```python
from build123d import *

# Parameters (mm, degrees)
BASE_FLANGE1_DEPTH           = 6.35
EDGE_FLANGE1_STRIP_W         = 41.3004
EDGE_FLANGE1_STRIP_H         = 6.35
EDGE_FLANGE1_STRIP_CUT_DEPTH = 520.7
EDGE_FLANGE1_DEPTH           = 520.7


# Sheet-metal steps are written as plain solids
with BuildPart() as part:
    # Sketch1 → Base-Flange1 (new body)
    with BuildSketch(Plane.XY):
        Polygon((-260.35, 127), (260.35, 127), (260.35, 46.0375), (269.875, 46.0375), (269.875, 20.6375), (260.35, 20.6375), (260.35, -112.7125), (269.875, -112.7125), (269.875, -138.1125), (215.9, -138.1125), (215.9, 0), (-215.9, 0), (-215.9, -138.1125), (-269.875, -138.1125), (-269.875, -112.7125), (-260.35, -112.7125), (-260.35, 20.6375), (-269.875, 20.6375), (-269.875, 46.0375), (-260.35, 46.0375), align=None)
    extrude(amount=-BASE_FLANGE1_DEPTH)

    # Edge-Flange1 strip (across the edge) → Edge-Flange1 strip cut (cut)
    with BuildSketch(Plane(origin=(260.35, 127, 0), x_dir=(0, -1, 0), z_dir=(-1, 0, 0))):
        with Locations((-6.35, -3.175)):
            Rectangle(EDGE_FLANGE1_STRIP_W, EDGE_FLANGE1_STRIP_H)
    extrude(amount=EDGE_FLANGE1_STRIP_CUT_DEPTH, mode=Mode.SUBTRACT)

    # Edge-Flange1 section (across the edge) → Edge-Flange1 (add)
    with BuildSketch(Plane(origin=(260.35, 127, 0), x_dir=(0, -1, 0), z_dir=(-1, 0, 0))):
        with BuildLine():
            Line((0, 7.9502), (0, 31.75))
            Line((0, 31.75), (6.35, 31.75))
            Line((6.35, 31.75), (6.35, 7.9502))
            ThreePointArc((6.35, 7.9502), (8.678559668, 2.328559668), (14.3002, 0))
            Line((14.3002, 0), (14.3002, -6.35))
            ThreePointArc((14.3002, -6.35), (4.188431608, -2.161568392), (0, 7.9502))
        make_face()
    extrude(amount=EDGE_FLANGE1_DEPTH)


solid = part.part
```
Build history of the part. All positions in model axes, mm. A direction names the side the tool comes from. Give positions to 0.01 mm unless a question says otherwise; leave off trailing zeros. Loops run counter-clockwise (first coordinate to the right, second up) from the corner with the lowest first, then second, coordinate; pieces in that order, holes last. Notation, with made-up numbers: (82.25, 51) -> (141.25, 51) arc R13 cw to (141.25, 61) -> close; hole circle Ø11 at (2.25, 72.25). An arc over 180 degrees is marked (long way). One line per question, with ' | ' between items. Start each with the question number.
1) 3-axis set-ups, long thin cutter, end or side, ignore diameter. For faces 1 (the flat face through (4, 120.65, 20)), 2 (the flat face through (-260.35, 98, -1)), 3 (the flat face through (260.35, 98, -1)): which of +Z, -Z, +X, -X, +Y, -Y reach the whole face in a straight line?
2) Cut at C-C (z = 14). Give the cut face in (x, y).
3) Probe L1, parallel to X at y = -104, z = -2; L2, parallel to Y at x = 79, z = 9; L3, parallel to Z at x = 117, y = 63. List the from-to ranges inside material, lowest first.
4) Cut at B-B (x = 13). Give the cut face in (y, z).
5) Cut at D-D (y = 33). Give the cut face in (x, z) (3 decimals).
6) Cut at A-A (y = -19). Give the cut face in (x, z), plus the area to 3 significant figures.
7) Two-plate mould, pull along Z, no slides. Class faces 4 (the flat face through (4, 45, -6.35)), 5 (the flat face through (4, 45, 0)), 6 (the flat face through (4, 127, 20)): released by +Z, released by -Z, zero draft, split by the parting line, or undercut.
8) Pin check, flat tips, straight feed: pin 1 (12 mm diameter, centred on x = 27, z = 14.5, fed in from -Y); pin 2 (3 mm diameter, centred on x = 267, z = -2, fed in from +Y); pin 3 (7 mm diameter, centred on x = 93, z = -2, fed in from -Y). Stop position of each tip, or through.
Return value:
1) face 1: +Z, +X, -X, -Y | face 2: +Z, -Z, -X, +Y | face 3: +Z, -Z, +X, +Y
2) outline: (-260.35, 120.65) -> (260.35, 120.65) -> (260.35, 127) -> (-260.35, 127) -> close
3) L1: -260.35 to -215.9, 215.9 to 260.35 | L2: 120.65 to 127 | L3: -6.35 to 0
4) outline: (0, -6.35) -> (112.7, -6.35) arc R14.3 ccw to (127, 7.95) -> (127, 31.75) -> (120.65, 31.75) -> (120.65, 7.95) arc R7.95 cw to (112.7, 0) -> (0, 0) -> close
5) outline: (-269.875, -6.35) -> (269.875, -6.35) -> (269.875, 0) -> (-269.875, 0) -> close
6) outline: (-260.35, -6.35) -> (-215.9, -6.35) -> (-215.9, 0) -> (-260.35, 0) -> close; (215.9, -6.35) -> (260.35, -6.35) -> (260.35, 0) -> (215.9, 0) -> close | area: 565 mm^2
7) face 4: released by -Z | face 5: released by +Z | face 6: zero draft
8) pin 1: y = 120.65 | pin 2: y = 46.04 | pin 3: y = 0
